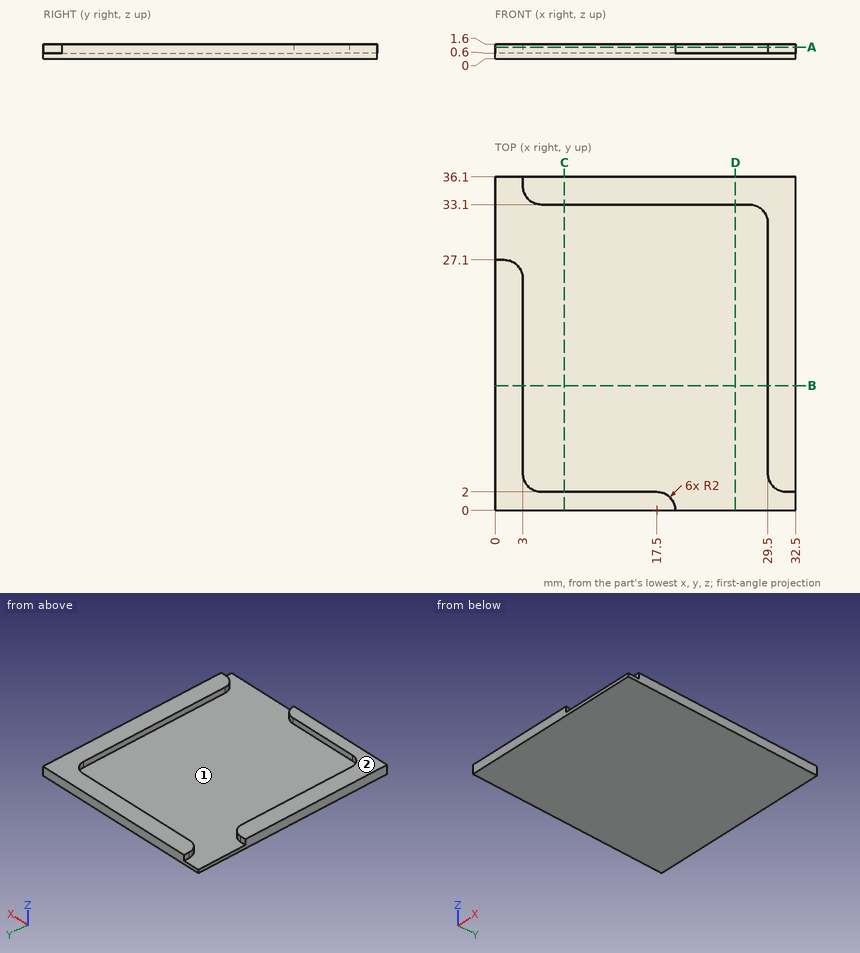
Input: dimensioned drawing with shaded views. Units: mm. Origin: part minimum x, y, z. Round coordinates to 2 decimals unless told otherwise and drop trailing zeros. Order: outer loops, then holes, each group sorted by start corner. A loop starts at its lowest first (then second) coordinate and runs counter-clockwise, first axis right, second up. Notation, with made-up numbers: (8.25, -16.5) - (57.25, -16.5) arc R19 cw to (57.25, 17.5) - close; hole circle Ø7 at (-8.75, 31.25). An arc over 180 degrees is marked (long way). Answer as a JSON object with one key per item and string values. Group by question number.
(1) Material intervals for probe 1 along Y at (x, z) = (17.5, 1.45); probe 2 along X at (y, z) = (12.5, 0.7); probe 3 along Z at (x, y) = (14.5, 21.5), sorted ascending. Write a range as from..to.
(2) Draft query along X for the marked faces 1 and 2. Return one class per face: released by +X, released by -X, zero draft, split by the parting line, or undercut.
(3) Cut plane A-A (z = 1.25). Return loops of the section in (x, y).
(4) Pin query (flat end, axial travel): P1, Ø8, axis at x = 28, y = 25, coming from the -Z side; P2, Ø0.8, axis at x = 0.5, z = 1.5, coming from the +Y side; P3, Ø10, axis at x = 18.5, y = 20, coming from the +Z side. Return the tip coordinate at first contact, or that it passes through.
(5) Cut plane C-C (x = 7.5). Return loops of the section in (y, z).
(6) Cut plane D-D (x = 26). Return loops of the section in (y, z), then the cut area to 3 significant figures.
(7) Cut plane B-B (y = 13.5). Return loops of the section in (x, z).
Here are the results:
{
 "1": {"probe 1": "y = 0..2, 33.1..36.1", "probe 2": "x = 0..3, 29.5..32.5", "probe 3": "z = 0..0.6"},
 "2": {"face 1": "undercut", "face 2": "zero draft"},
 "3": {"outline": "(0, 0) - (19.5, 0) arc R2 ccw to (17.5, 2) - (5, 2) arc R2 cw to (3, 4) - (3, 25.1) arc R2 ccw to (1, 27.1) - (0, 27.1) - close; (3, 35.1) arc R2 ccw to (5, 33.1) - (27.5, 33.1) arc R2 cw to (29.5, 31.1) - (29.5, 4) arc R2 ccw to (31.5, 2) - (32.5, 2) - (32.5, 36.1) - (3, 36.1) - close"},
 "4": {"P1": "stops at z = 0", "P2": "stops at y = 27.1", "P3": "stops at z = 0.6"},
 "5": {"outline": "(0, 0) - (36.1, 0) - (36.1, 1.6) - (33.1, 1.6) - (33.1, 0.6) - (2, 0.6) - (2, 1.6) - (0, 1.6) - close"},
 "6": {"outline": "(0, 0) - (36.1, 0) - (36.1, 1.6) - (33.1, 1.6) - (33.1, 0.6) - (0, 0.6) - close", "area": "24.7 mm^2"},
 "7": {"outline": "(0, 0) - (32.5, 0) - (32.5, 1.6) - (29.5, 1.6) - (29.5, 0.6) - (3, 0.6) - (3, 1.6) - (0, 1.6) - close"}
}
